Check sheet for the drawn part. Datum: minimum x, y, z corner. Units: mm. Round coordinates to 2 decimals unless told otherwise and drop trailing zeros. Write each loop counter-clockwise with the first axis right and the second up, starting at its lowest first coordinate (ties: lowest second). Pieces come first, ordered by that corner, then holes. Notation, with made-up numbers: (-3, 36.25) - (43, 36.25) arc R13 cw to (43, 55.25) - close; hole circle Ø1 at (14.5, 29.5). An arc over 180 degrees is marked (long way). Write each question's results on one line, items separated by ' | '.
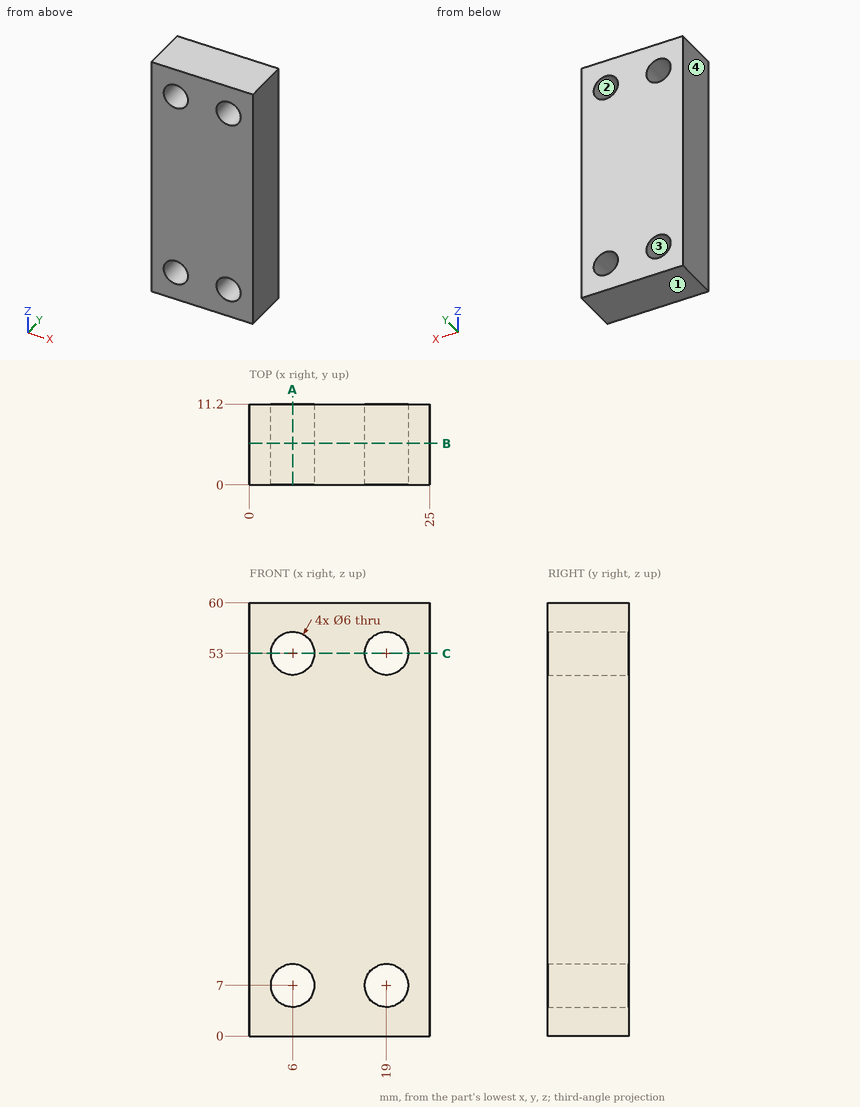
(1) Section check A-A (x = 6). Record the cut outline in (y, z), plus the area to 3 significant figures.
Answer:
outline: (0, 0) - (11.2, 0) - (11.2, 4) - (0, 4) - close; (0, 10) - (11.2, 10) - (11.2, 50) - (0, 50) - close; (0, 56) - (11.2, 56) - (11.2, 60) - (0, 60) - close | area: 538 mm2
(2) Mould release check, pull along Z, two halves, no side actions. Record for the marked faces 1, 2, 3 and 4: released by +Z, released by -Z, zero draft, split by the parting line, or undercut.
Answer:
face 1: released by -Z | face 2: undercut | face 3: undercut | face 4: zero draft
(3) Section check C-C (z = 53). Record the cut outline in (x, y), plus the area to 3 significant figures.
Answer:
outline: (0, 0) - (3, 0) - (3, 11.2) - (0, 11.2) - close; (9, 0) - (16, 0) - (16, 11.2) - (9, 11.2) - close; (22, 0) - (25, 0) - (25, 11.2) - (22, 11.2) - close | area: 146 mm2
(4) Section check B-B (y = 5.75). Record the cut outline in (x, z).
Answer:
outline: (0, 0) - (25, 0) - (25, 60) - (0, 60) - close; hole circle Ø6 at (6, 7); hole circle Ø6 at (6, 53); hole circle Ø6 at (19, 7); hole circle Ø6 at (19, 53)
(5) Thickness scan on L1, parallel to X at y = 6.5, z = 7; L2, parallel to Z at x = 19, y = 4.5; L3, parallel to Z at x = 3.75, y = 2. Record the ranges inside material, lowest first.
Answer:
L1: 0 to 3, 9 to 16, 22 to 25 | L2: 0 to 4, 10 to 50, 56 to 60 | L3: 0 to 5.02, 8.98 to 51.02, 54.98 to 60
